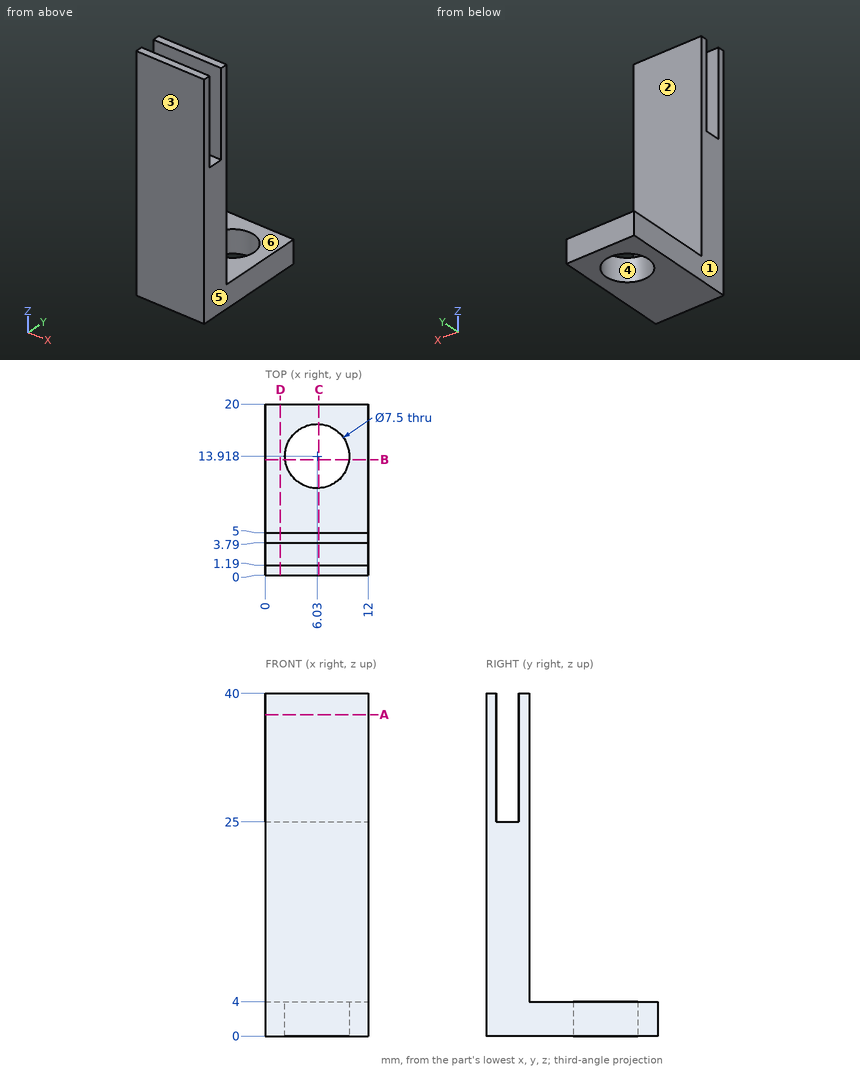
Design review of the part shown in the three views and the two pictorial views. Dimensions are in mm from the part's minimum x, y and z. A direction names the side the tool comes from. Give positions to 0.01 mm unless a question says otherwise; leave off trailing zeros. Order: outer loops, then holes, each group sorted by start corner. A loop starts at its lowest first (then second) coordinate and runs counter-clockwise, first axis right, second up. Notation, with made-up numbers: (-32, 83) -> (-25, 83) arc R17 cw to (-25, 114) -> close; hole circle Ø5 at (24.25, 80.5). An arc over 180 degrees is marked (long way). Write each question's results on one line, items separated by ' | '. Start each with the question number.
Q1. For pin 1 (1.3 mm diameter, centred on x = 7.5, y = 2.5, fed in from +Z); pin 2 (1.5 mm diameter, centred on x = 7, y = 17, fed in from +Z); pin 3 (7 mm diameter, centred on x = 6.03, y = 13.92, fed in from -Z); pin 4 (2 mm diameter, centred on x = 6, z = 35, fed in from +Y), all flat-tipped, find the tip position at first contact; note any pin that passes through.
Q2. Add section A-A on z = 37.5. Give the boundary of the cut face in (x, y), and give its area (3 significant figures).
Q3. Add section D-D on x = 1.75. Give the boundary of the cut face in (y, z), and give its area (3 significant figures).
Q4. Add section C-C on x = 6.25. Give the boundary of the cut face in (y, z) (1 decimal), and give its area (3 significant figures).
Q5. Machinability: for the marked faces 5 and 6, which of the approach directions +Z, -Z, +X, -X, +Y, -Y give a long, thin tool a straight path to every point of the face, cutting with its end or side? Answer none if there is none.
Q6. Wall thickness on L1, parallel to Y at x = 4.75, z = 32; L2, parallel to Z at x = 1.25, y = 13; L3, parallel to Y at x = 4.5, z = 20: over which ranges is each line inside the solid? List them lowest first. Write a range as from..to.
Q7. Mouldability with a two-part tool opening along Y and no side actions: class the marked faces 1, 2, 3 and 4 as +Y half, -Y half, draft (parallel to the pull), parting line (faces both ways), or undercut.
Q8. Add section B-B on y = 13.5. Give the boundary of the cut face in (x, z).
Found:
1) pin 1: stops at z = 25 | pin 2: stops at z = 4 | pin 3: passes through | pin 4: stops at y = 5
2) outline: (0, 0) -> (12, 0) -> (12, 1.19) -> (0, 1.19) -> close; (0, 3.79) -> (12, 3.79) -> (12, 5) -> (0, 5) -> close | area: 28.8 mm2
3) outline: (0, 0) -> (20, 0) -> (20, 4) -> (5, 4) -> (5, 40) -> (3.79, 40) -> (3.79, 25) -> (1.19, 25) -> (1.19, 40) -> (0, 40) -> close | area: 221 mm2
4) outline: (0, 0) -> (10.2, 0) -> (10.2, 4) -> (5, 4) -> (5, 40) -> (3.8, 40) -> (3.8, 25) -> (1.2, 25) -> (1.2, 40) -> (0, 40) -> close; (17.7, 0) -> (20, 0) -> (20, 4) -> (17.7, 4) -> close | area: 191 mm2
5) face 5: +Z, -Z, +X, +Y, -Y | face 6: +Z, +X, -X, +Y
6) L1: y = 0..1.19, 3.79..5 | L2: z = 0..4 | L3: y = 0..5
7) face 1: draft | face 2: +Y half | face 3: -Y half | face 4: undercut
8) outline: (0, 0) -> (2.3, 0) -> (2.3, 4) -> (0, 4) -> close; (9.76, 0) -> (12, 0) -> (12, 4) -> (9.76, 4) -> close
